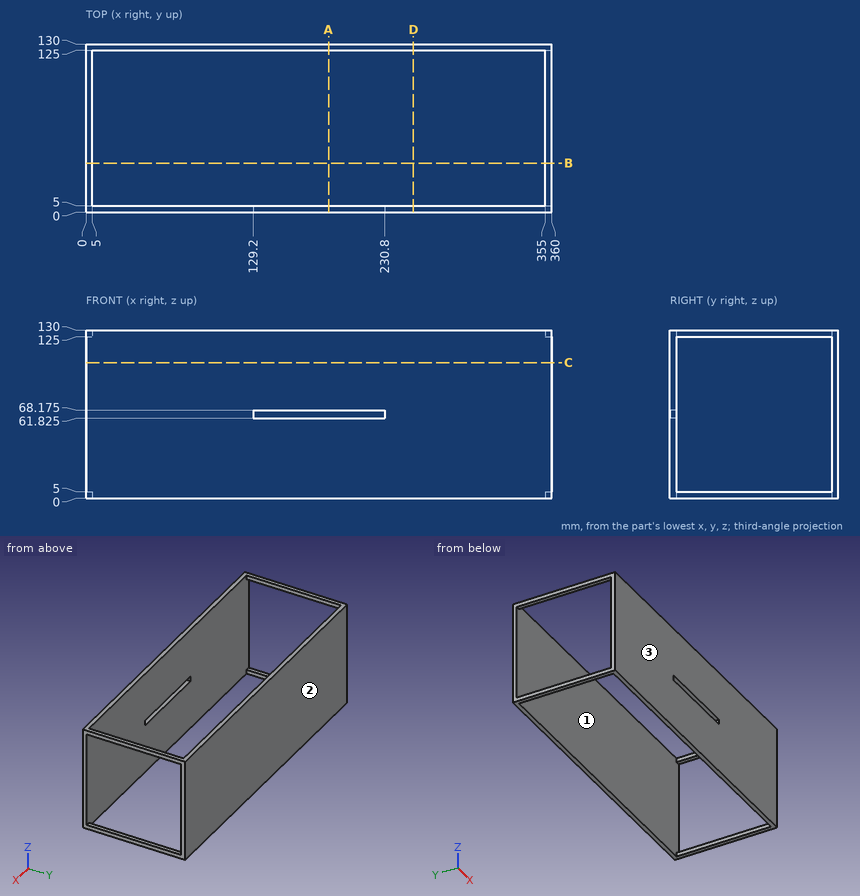
Check sheet for the drawn part. Datum: minimum x, y, z corner. Units: mm. Round coordinates to 2 decimals unless told otherwise and drop trailing zeros. Write each loop counter-clockwise with the first axis right and the second up, starting at its lowest first coordinate (ties: lowest second). Pieces come first, ordered by that corner, then holes. Notation, with made-up numbers: (32.25, 47.25) -> (79.25, 47.25) arc R14 cw to (79.25, 70.25) -> close; hole circle Ø3 at (-9.75, -30.5). An arc over 180 degrees is marked (long way). Write each question's results on one line, items separated by ' | '. Start each with the question number.
1. Cross-section at B-B (y = 38). Enter the section's corners in (x, z).
2. Cross-section at A-A (x = 187.5). Enter the section's corners in (y, z) (3 decimals), then the cut area to 3 significant figures.
3. Cross-section at C-C (z = 105). Enter the section's corners in (x, y), then the cut area to 3 significant figures.
4. Draft check along Y on the marked faces 1, 2 and 3. Enter one of: +Y half, -Y half, draft (parallel to the pull), parting line (faces both ways), or undercut.
5. Cross-section at D-D (x = 253). Enter the section's corners in (y, z), then the cut area to 3 significant figures.
6. Material ranges on probe 1 along Y at (x, z) = (16, 41.5), recorded low to high. Write a range as from..to.
7. Depth check by flat-ended pin: P1, Ø2, axis at x = 242, z = 111, coming from the -Y side. Enter the tip coordinate at first touch or a pass-through.
Solutions:
1) outline: (0, 0) -> (5, 0) -> (5, 5) -> (0, 5) -> close; (0, 125) -> (5, 125) -> (5, 130) -> (0, 130) -> close; (355, 0) -> (360, 0) -> (360, 5) -> (355, 5) -> close; (355, 125) -> (360, 125) -> (360, 130) -> (355, 130) -> close
2) outline: (0, 0) -> (5, 0) -> (5, 61.825) -> (0, 61.825) -> close; (0, 68.175) -> (5, 68.175) -> (5, 130) -> (0, 130) -> close; (125, 0) -> (130, 0) -> (130, 130) -> (125, 130) -> close | area: 1,270 mm2
3) outline: (0, 0) -> (360, 0) -> (360, 5) -> (0, 5) -> close; (0, 125) -> (360, 125) -> (360, 130) -> (0, 130) -> close | area: 3,600 mm2
4) face 1: undercut | face 2: +Y half | face 3: -Y half
5) outline: (0, 0) -> (5, 0) -> (5, 130) -> (0, 130) -> close; (125, 0) -> (130, 0) -> (130, 130) -> (125, 130) -> close | area: 1,300 mm2
6) probe 1: y = 0..5, 125..130
7) P1: stops at y = 0
